Here's how the part is built. I have some questions about the finished solid (model axes, mm). Coordinates: 2 decimals unless noted, no trailing zeros. Loops run counter-clockwise (first coordinate to the right, second up) from the corner with the lowest first, then second, coordinate; pieces in that order, holes last.
```python
from build123d import *

# Parameters (mm, degrees)
SKETCH2_W               = 431.8
SKETCH2_H               = 127
BOSS_EXTRUDE1_DEPTH     = 3.175
CUT_EXTRUDE1_DEPTH      = 451.100345062
CUT_EXTRUDE1_DEPTH_BACK = 451.100345062
CUT_EXTRUDE2_DEPTH      = 451.100345062
CUT_EXTRUDE2_DEPTH_BACK = 451.100345062


with BuildPart() as part:
    # Sketch2 → Boss-Extrude1 (new body)
    with BuildSketch(Plane.XY):
        with Locations((215.9, 63.5)):
            Rectangle(SKETCH2_W, SKETCH2_H)
    extrude(amount=BOSS_EXTRUDE1_DEPTH)

    # Sketch3 → Cut-Extrude1 (cut, two sides: drawn at the far end of the back side and taken through both)
    with BuildSketch(Plane.ZY.offset(-CUT_EXTRUDE1_DEPTH_BACK)):
        Polygon((-132.039681301, -228.699436628), (0, 0), (3.175, 5.499261314), (135.214681301, 234.198697942), (592.613554557, -29.880664659), (325.359191955, -492.77879923), align=None)
    extrude(amount=CUT_EXTRUDE1_DEPTH + CUT_EXTRUDE1_DEPTH_BACK, mode=Mode.SUBTRACT)

    # Sketch4 → Cut-Extrude2 (cut, two sides: drawn at the far end of the back side and taken through both)
    with BuildSketch(Plane(origin=(431.8, 0, 0), x_dir=(0, 0, -1), z_dir=(1, 0, 0)).offset(-CUT_EXTRUDE2_DEPTH_BACK)):
        Polygon((228.699436628, 259.039681301), (0, 127), (-3.175, 125.166912895), (-231.874436628, -6.872768405), (-495.95379923, 450.526104851), (-35.379925973, 716.438554557), align=None)
    extrude(amount=CUT_EXTRUDE2_DEPTH + CUT_EXTRUDE2_DEPTH_BACK, mode=Mode.SUBTRACT)


solid = part.part
```
1. I want a section at B-B (z = 1.15). Please give me the cut outline in (x, y), then the cut area to 3 significant figures.
2. For pin 1 (1.5 mm diameter, centred on x = 55.5, z = 1.5, fed in from -Y), with a flat end and sliding along its axis, tell me the tip position at first contact or that it passes through.
3. I need wall thicknesses on line 1 along Y through (x, z) = (159.5, 1.25); line 2 along Y through (x, z) = (350.5, 2.8). Which ranges of each line are inside material? Lowest first, please.
4. I want a section at A-A (x = 364.5). Please give me the cut outline in (y, z) (3 decimals).
Response values:
1. outline: (0, 1.99) - (431.8, 1.99) - (431.8, 126.34) - (0, 126.34) - close
1. area: 53,700 mm2
2. pin 1: stops at y = 1.3
3. line 1: y = 2.17 to 126.28
3. line 2: y = 4.85 to 125.38
4. outline: (0, 0) - (127, 0) - (125.167, 3.175) - (5.499, 3.175) - close
